Can you work these out from the drawing? Everything is in mm from the part's minimum corner. Coordinates: 2 decimals unless noted, no trailing zeros. Loops run counter-clockwise (first coordinate to the right, second up) from the corner with the lowest first, then second, coordinate; pieces in that order, holes last. Notation, with made-up numbers: (-2.5, 11) -> (2.5, 11) arc R25 cw to (2.5, 26) -> close; hole circle Ø5 at (55, 20). An arc over 180 degrees is marked (long way). One line per question, with ' | ' between items.
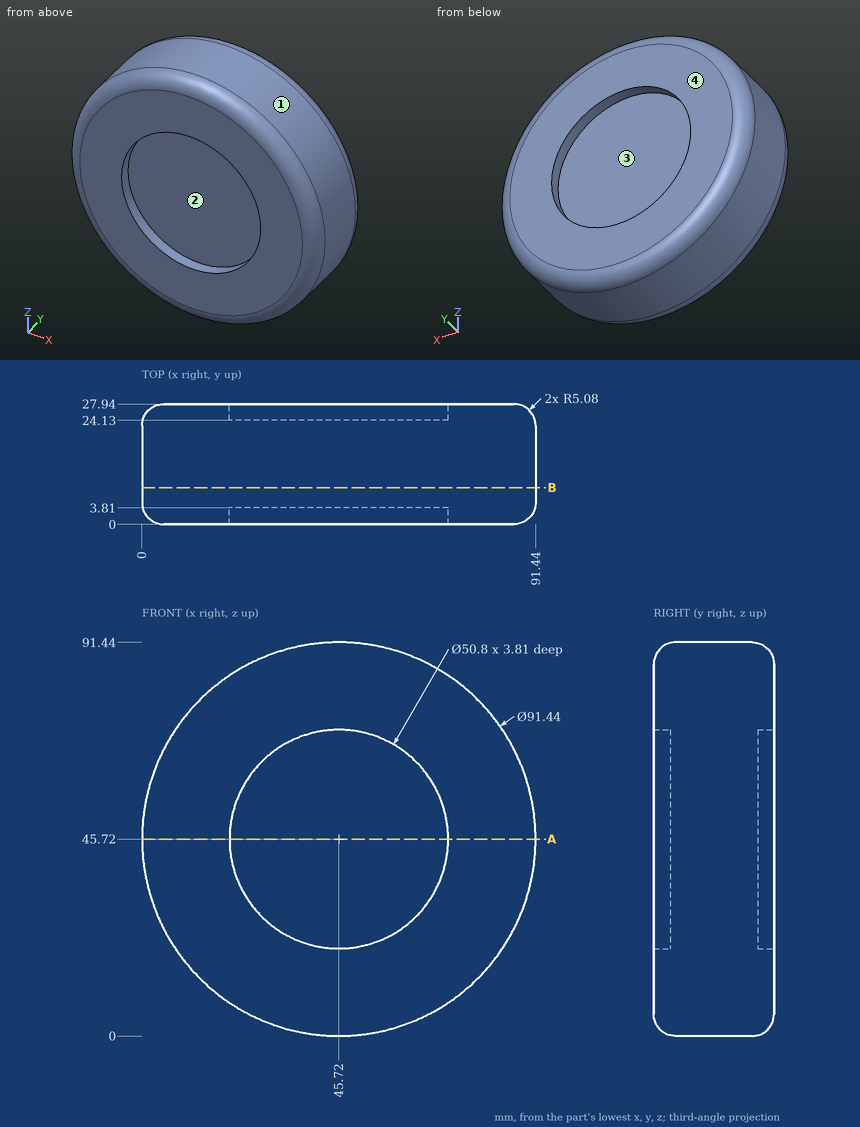
Q1. For pin 1 (10 mm diameter, centred on x = 78.5, z = 12.5, fed in from -Y); pin 2 (6 mm diameter, centred on y = 8, z = 39.5, fed in from -X); pin 3 (12 mm diameter, centred on x = 66.5, y = 11.5, fed in from -Z), each with a flat end and sliding along its axis, tell me the tip position at first contact or that it passes through.
Values follow:
pin 1: stops at y = 0.11 | pin 2: stops at x = 0.11 | pin 3: stops at z = 2.45
Q2. Imagine slicing it at B-B on y = 8.5. Write out the boundary of the cut face in (x, z).
Values follow:
outline: circle Ø91.44 at (45.72, 45.72)
Q3. Imagine slicing it at A-A on z = 45.72. Write out the boundary of the cut face in (x, y), plus the area to 3 significant figures.
Values follow:
outline: (0, 5.08) arc R5.08 ccw to (5.08, 0) -> (20.32, 0) -> (20.32, 3.81) -> (71.12, 3.81) -> (71.12, 0) -> (86.36, 0) arc R5.08 ccw to (91.44, 5.08) -> (91.44, 22.86) arc R5.08 ccw to (86.36, 27.94) -> (71.12, 27.94) -> (71.12, 24.13) -> (20.32, 24.13) -> (20.32, 27.94) -> (5.08, 27.94) arc R5.08 ccw to (0, 22.86) -> close | area: 2,150 mm2
Q4. Please list where these lines run through material, in increasing order: L1, parallel to Z at x = 45.72, y = 25.85; L2, parallel to Z at x = 45.72, y = 3.05; L3, parallel to Y at x = 28, z = 45.5. Write a range as [from, to].
Values follow:
L1: z = [0.97, 20.32], [71.12, 90.47] | L2: z = [0.42, 20.32], [71.12, 91.02] | L3: y = [3.81, 24.13]
Q5. We'd pull the mould along X, two halves only. Please class the marked faces 1, 2, 3 and 4: released by +X, released by -X, zero draft, split by the parting line, or undercut.
Values follow:
face 1: split by the parting line | face 2: undercut | face 3: undercut | face 4: zero draft
